Geometry: final body of the model. Coordinates: model frame, mm. A direction names the side the tool comes from. Give positions to 0.01 mm unless a question says otherwise; leave off trailing zeros. Loops run counter-clockwise (first coordinate to the right, second up) from the corner with the lowest first, then second, coordinate; pieces in that order, holes last. Notation, with made-up numbers: M 4.25,70.25 L 53.25,70.25 A17 ccw 53.25,101.25 Z; hole C 0.5,65 d6. An arc over 180 degrees is marked long. Put each result on its own line as item: value.
```python
from build123d import *

# Parameters (mm, degrees)
EXTRUDE_1_DEPTH = 2
EXTRUDE_2_DEPTH = 2.5


with BuildPart() as part:
    # 草图1 → 凸台-拉伸1 (new body)
    with BuildSketch(Plane(origin=(0, 0, 0), x_dir=(1, 0, 0), z_dir=(0, 1, 0))):
        Polygon((-1.25, 32), (-1.25, -32), (81.25, -32), (83.75, -41.313840204), (159.893914202, -96.432841737), (208.269633633, -29.6044064), (193.688884105, -19.049703979), (182.840995505, -34.035474327), (121.277830831, 10.528824785), (83.75, 32), align=None)
        Polygon((0, 30.75), (0, -30.75), (82.208724754, -30.75), (84.842274477, -40.561384515), (159.614327597, -94.687324241), (206.524116136, -29.883993005), (193.968470709, -20.795221475), (183.12058211, -35.780991824), (120.599033271, 9.477061724), (83.417685679, 30.75), align=None, mode=Mode.SUBTRACT)
    extrude(amount=-EXTRUDE_1_DEPTH)

    # 草图2 → 凸台-拉伸2 (add)
    with BuildSketch(Plane(origin=(0, 0, 0), x_dir=(1, 0, 0), z_dir=(0, 1, 0))):
        Polygon((-1.25, 32), (-1.25, -32), (81.25, -32), (83.75, -41.313840204), (159.893914202, -96.432841737), (208.269633633, -29.6044064), (193.688884105, -19.049703979), (182.840995505, -34.035474327), (121.277830831, 10.528824785), (83.75, 32), align=None)
    extrude(amount=EXTRUDE_2_DEPTH)


solid = part.part
```
Item 1: Set-up query: faces 4 (the flat face through (111, -2, 60)), 5 (the flat face through (188.62, -0.986, 28.183)), 6 (the flat face through (152.49, 0.219, 12.065)). Return all of +Z, -Z, +X, -X, +Y, -Y with unobstructed straight access to the full face (end or side cutting, diameter ignored); none if empty.
Output values:
face 4: +Z, -Z, +X, -X, -Y
face 5: -Y
face 6: -Z, +Y, -Y
Item 2: Section B-B on x = 47. Output: boundary loops of the cut face in (y, z), then the cut area to 3 significant figures.
Output values:
outline: M -2,-32 L 2.5,-32 L 2.5,32 L -2,32 L -2,30.75 L 0,30.75 L 0,-30.75 L -2,-30.75 Z
area: 165 mm²
Item 3: Pin query (flat end, axial travel): pin 1 Ø1.5 at (y, z) = (-0.5, 64.5) entering from -X; pin 2 Ø1.5 at (x, y) = (143.5, 1) entering from -Z; pin 3 Ø0.6 at (x, y) = (45, -0.5) entering from +Z. Return the tip coordinate at first contact, or that it passes through.
Output values:
pin 1: x = 114.74
pin 2: z = 5.01
pin 3: z = 32
Item 4: Section C-C on z = 65. Output: boundary loops of the cut face in (x, y), then the cut area to 3 significant figures.
Output values:
outline: M 116.47,-2 L 118.6,-2 L 118.6,0 L 181.1,0 L 181.1,-2 L 182.65,-2 L 182.65,2.5 L 116.47,2.5 Z
area: 173 mm²
Item 5: Line query: probe 1 along X at (y, z) = (-0.3, 23); probe 2 along Y at (x, z) = (80, -26); probe 3 along Z at (x, y) = (26.5, 2.2). Output: solid intervals per line, ascending. Write a range as [from, to].
Output values:
probe 1: [-1.25, 0], [165.46, 167.6], [190.83, 192.37], [197.01, 199.15]
probe 2: [0, 2.5]
probe 3: [-32, 32]
Item 6: Section A-A on y = -0.75. Output: boundary loops of the cut face in (x, z).
Output values:
outline: M -1.25,-32 L 83.75,-32 L 121.28,-10.53 L 182.84,34.04 L 193.69,19.05 L 208.27,29.6 L 159.89,96.43 L 83.75,41.31 L 81.25,32 L -1.25,32 Z; hole M 0,-30.75 L 83.42,-30.75 L 120.6,-9.48 L 183.12,35.78 L 193.97,20.8 L 206.52,29.88 L 159.61,94.69 L 84.84,40.56 L 82.21,30.75 L 0,30.75 Z
Item 7: Mould query, pull axis Z, two halves, no side actions, for faces 1 (the flat face through (102.8, 0.2, -21.1)), 2 (the flat face through (39, 0, 32)), 3 (the flat face through (121.705, -0.986, 67.245)). Classes: pulls with the +Z half, pulls with the -Z half, needs draft (parallel to the pull), parting line crosses it, or undercut.
Output values:
face 1: pulls with the -Z half
face 2: pulls with the +Z half
face 3: undercut
